Design review of the part built by this model. Coordinates are the model's own, in mm. A direction names the side the tool comes from. Round coordinates to 2 decimals unless told otherwise and drop trailing zeros. Write each loop counter-clockwise with the first axis right and the second up, starting at its lowest first coordinate (ties: lowest second). Pieces come first, ordered by that corner, then holes. Notation, with made-up numbers: M -26.75,36 L -3.75,36 A12 cw -3.75,56 Z; hole C 50.5,52 d1. An arc over 180 degrees is marked long. Use CSV: the item, a comma, the result in double quotes.
Autodesk Inventor part; units mm, degrees
ref_plane "YZ Plane" through (0, 0, 0) normal (1, 0, 0) x (0, 1, 0)
ref_plane "XZ Plane" through (0, 0, 0) normal (0, 1, 0) x (-1, 0, 0)
ref_plane "XY Plane" through (0, 0, 0) normal (0, 0, 1) x (1, 0, 0)
sketch "Sketch1" plane through (0, 0, 0) normal (0, 1, 0) x (-1, 0, 0)
  line L0 (-15, -15) -> (15, -15)
  line L1 (15, -15) -> (15, 15)
  line L2 (15, 15) -> (-15, 15)
  line L3 (-15, 15) -> (-15, -15)
  line L4 (-15, -15) -> (15, 15) construction
  line L5 (15, -15) -> (-15, 15) construction
  point P0 (0, 0)
  dimension "d0" = 30
  dimension "d1" = 30
extrude "Extrusion1" add sketch "Sketch1" along normal blind 21
sketch "Sketch2" plane through (15, 0, 15) normal (1, 0, 0) x (0, 0, -1)
  circle A0 centre (15, 10.5) radius 8
  line L0 (0, 21) -> (30, 21)
  point P0 (15, 0)
  point P1 (15, 21)
  dimension "d4" = 16
  dimension "d29" = 10.5
extrude "Extrusion2" add sketch "Sketch2" along normal blind 57
sketch "Sketch3" plane through (0, 21, 0) normal (0, 1, 0) x (1, 0, 0)
  circle A0 centre (37, 0) radius 2.5
  circle A1 centre (57, 0) radius 2.5
  line L0 (15, -15) -> (15, 15)
  line L1 (72, -8) -> (72, 8)
  circle A2 centre (10, -10) radius 2.5
  line L2 (1.0234, -33.583) -> (-6.5136, -33.583)
  line L3 (-6.5136, -33.583) -> (-6.5136, -27.1544)
  circle A3 centre (-10, -10) radius 2.5
  circle A4 centre (10, 10) radius 2.5
  circle A5 centre (-10, 10) radius 2.5
  line L4 (-15, -15) -> (15, -15)
  line L5 (-15, 15) -> (-15, -15)
  point P0 (0, 0)
  point P1 (15, 0)
  point P2 (72, 0)
  dimension "d7" = 5
  dimension "d8" = 5
  dimension "d9" = 22
  dimension "d10" = 20
  dimension "d12" = 5
  dimension "d15" = 20
  dimension "d18" = 20
  dimension "d21" = 5
  dimension "d22" = 5
  dimension "d28" = 15
chamfer "Chamfer1" distance 2.5 angle 45 1 edges at (15, 10.5, 8)
extrude "Extrusion4" cut sketch "Sketch3" against normal through all contours A2 | A3 | A4 | A5
extrude "Extrusion5" cut sketch "Sketch3" against normal through all contours A0 | A1
properties part number "RodConnector_3DPrint"
1) For pin 1 Ø4 at (x, z) = (37, 0) entering from -Y; pin 2 Ø1 at (x, y) = (39.5, 12) entering from +Z; pin 3 Ø5 at (x, z) = (38.5, 4) entering from -Y; pin 4 Ø6 at (x, y) = (53, 13.5) entering from -Z, all flat-tipped, find the tip position at first contact; note any pin that passes through.
Answers:
pin 1,"through"
pin 2,"z = 7.94"
pin 3,"y = 2.65"
pin 4,"z = -8"
2) Add section D-D on x = 33.5. Write out the cut boundary in (y, z), then the cut area to 3 significant figures.
Answers:
outline,"C 10.5,0 d16"
area,"201 mm²"
3) Add section C-C on x = -10. Write out the cut boundary in (y, z), then the cut area to 3 significant figures.
Answers:
outline,"M 0,-15 L 21,-15 L 21,-12.5 L 0,-12.5 Z; M 0,-7.5 L 21,-7.5 L 21,7.5 L 0,7.5 Z; M 0,12.5 L 21,12.5 L 21,15 L 0,15 Z"
area,"420 mm²"
4) Wall thickness on line 1 along Z through (x, y) = (-10, 13.5); line 2 along X through (y, z) = (15, -0.25): over which ranges is each line inside the solid? List them lowest first. Write a range as [from, to].
Answers:
line 1,"[-15, -12.5], [-7.5, 7.5], [12.5, 15]"
line 2,"[-15, 34.51], [39.49, 54.51], [59.49, 72]"
5) The part is to be moulded in two halves that separate along Z. For faces 1 (the face through (-10.54, 10.65, 12.44)), 2 (the face through (44.37, 13.56, -7.39)), 3 (the face through (0, 10, 15)), say which applies: released by +Z, released by -Z, zero draft, split by the parting line, or undercut.
Answers:
face 1,"undercut"
face 2,"split by the parting line"
face 3,"released by +Z"
6) Add section A-A on z = 0. Give the number of separate pieces and of enclosed holes in the cut face, then the cut area to 3 significant figures.
Answers:
separate pieces,"3"
enclosed holes,"0"
area,"1,390 mm²"
7) Machinability: for faces 4 (the face through (15, 6, 10)), 5 (the face through (0, 0, 0)), which of the approach directions +Z, -Z, +X, -X, +Y, -Y give a long, thin tool a straight path to every point of the face, cutting with its end or side? Answer none if there is none.
Answers:
face 4,"+X"
face 5,"+Z, -Z, +X, -X, -Y"
8) Add section B-B on y = 10.5. Write out the cut boundary in (x, z), then the cut area to 3 significant figures.
Answers:
outline,"M -15,-15 L 15,-15 L 15,-10.5 L 17.5,-8 L 72,-8 L 72,8 L 17.5,8 L 15,10.5 L 15,15 L -15,15 Z; hole C -10,-10 d5; hole C -10,10 d5; hole C 10,-10 d5; hole C 10,10 d5; hole C 37,0 d5; hole C 57,0 d5"
area,"1,700 mm²"
